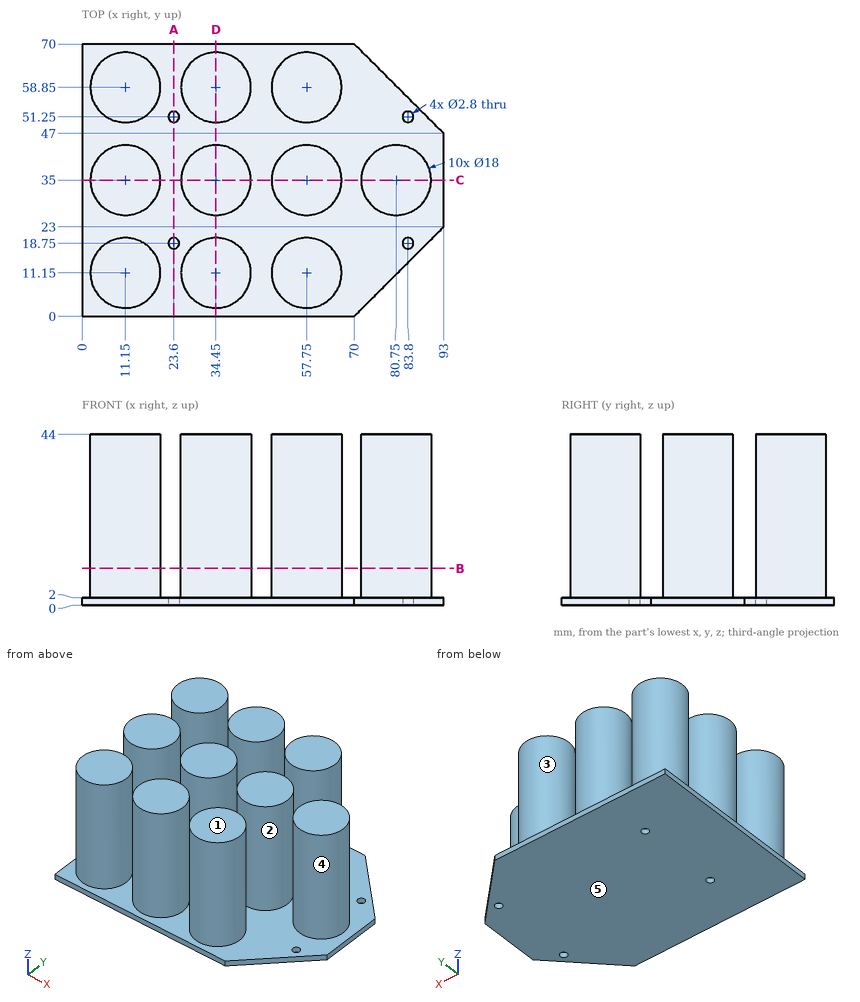
Here's the drawing with two shaded views (mm, measured from the low corner). I have some questions. A direction names the side the tool comes from. Give positions to 0.01 mm unless a question says otherwise; leave off trailing zeros. Loops run counter-clockwise (first coordinate to the right, second up) from the corner with the lowest first, then second, coordinate; pieces in that order, holes last. Notation, with made-up numbers: (-29.75, -23) -> (-9.75, -23) arc R18 ccw to (-9.75, -3) -> close; hole circle Ø6 at (-33.5, -8.5). An arc over 180 degrees is marked (long way). Answer as a JSON object with one key per item and string values. Group by question number.
Item 1: Imagine slicing it at A-A on x = 23.6. Write out the boundary of the cut face in (y, z), then the cut area to 3 significant figures.
Item 2: Imagine slicing it at C-C on y = 35. Write out the boundary of the cut face in (x, z).
Item 3: Imagine slicing it at D-D on x = 34.45. Write out the boundary of the cut face in (y, z), then the cut area to 3 significant figures.
Item 4: Imagine slicing it at B-B on z = 9.5. Give the number of separate pieces and of enclosed holes in the cut face, then the cut area to 3 significant figures.
Item 5: Thinking about a two-plate mould opening in Y: for the marked faces 3, 4 and 5, which applies, pulls with the +Y half, pulls with the -Y half, needs draft (parallel to the pull), parting line crosses it, or undercut?
Item 6: I need wall thicknesses on L1, parallel to Y at x = 32.5, z = 29; L2, parallel to Y at x = 23.6, z = 1.55; L3, parallel to X at y = 51, z = 5. Which ranges of each line are inside material? Lowest first, please.
Item 7: Will these pins go through, and if not, where does the flat tip stop? pin 1 (8 mm diameter, centred on y = 49.5, z = 38, fed in from +X); pin 2 (1.7 mm diameter, centred on x = 83.8, y = 18.75, fed in from +Z); pin 3 (1 mm diameter, centred on x = 51.5, z = 6.5, fed in from +Y); pin 4 (1.5 mm diameter, centred on y = 17, z = 33.5, fed in from -X).
Item 8: On a 3-axis mill with a long thin cutter (end or side, diameter ignored), from which of +Z, -Z, +X, -X, +Y, -Y can I reach the whole of each face in a straight line? I mean the marked faces 1 and 2. Say none if no direction works.
Answer list:
{
 "1": {"outline": "(0, 0) -> (17.35, 0) -> (17.35, 2) -> (0, 2) -> close; (20.15, 0) -> (49.85, 0) -> (49.85, 2) -> (20.15, 2) -> close; (52.65, 0) -> (70, 0) -> (70, 2) -> (52.65, 2) -> close", "area": "129 mm2"},
 "2": {"outline": "(0, 0) -> (93, 0) -> (93, 2) -> (89.75, 2) -> (89.75, 44) -> (71.75, 44) -> (71.75, 2) -> (66.75, 2) -> (66.75, 44) -> (48.75, 44) -> (48.75, 2) -> (43.45, 2) -> (43.45, 44) -> (25.45, 44) -> (25.45, 2) -> (20.15, 2) -> (20.15, 44) -> (2.15, 44) -> (2.15, 2) -> (0, 2) -> close"},
 "3": {"outline": "(0, 0) -> (70, 0) -> (70, 2) -> (67.85, 2) -> (67.85, 44) -> (49.85, 44) -> (49.85, 2) -> (44, 2) -> (44, 44) -> (26, 44) -> (26, 2) -> (20.15, 2) -> (20.15, 44) -> (2.15, 44) -> (2.15, 2) -> (0, 2) -> close", "area": "2,410 mm2"},
 "4": {"separate pieces": "10", "enclosed holes": "0", "area": "2,540 mm2"},
 "5": {"face 3": "undercut", "face 4": "parting line crosses it", "face 5": "needs draft"},
 "6": {"L1": "y = 2.36 to 19.94, 26.21 to 43.79, 50.06 to 67.64", "L2": "y = 0 to 17.35, 20.15 to 49.85, 52.65 to 70", "L3": "x = 6.75 to 15.55, 30.05 to 38.85, 53.35 to 62.15"},
 "7": {"pin 1": "stops at x = 64.99", "pin 2": "passes through", "pin 3": "stops at y = 65.77", "pin 4": "stops at x = 3.73"},
 "8": {"face 1": "+Z, +X, -X, +Y, -Y", "face 2": "+Z"}
}
